Could you check a few things on this model? Use its own coordinates, in mm. A direction names the side the tool comes from. Coordinates: 2 decimals unless noted, no trailing zeros. Order: outer loops, then holes, each group sorted by start corner. A loop starts at its lowest first (then second) coordinate and runs counter-clockwise, first axis right, second up. Notation, with made-up numbers: (-8, -32) -> (0, -32) arc R25 ccw to (0, -14) -> close; hole circle Ø2 at (27.5, 2). An arc over 180 degrees is marked (long way). Use a Markdown table: item, result. Add a question column.
1) If we section it at B-B (z = -1.5): Write out the boundary of the cut face in (x, y).
2) If we section it at D-D (y = 1): Give the number of separate pieces and of enclosed holes in the cut face, plus the area to 3 significant figures.
3) Which directions (+Z, -Z, +X, -X, +Y, -Y) give clear straight access to the entire face, cutting with the end or side of a thin tool? Please do faces 1 (the flat face through (-69, 0, -35)), 2 (the flat face through (-49.5, 0, 15.3)), 3 (the flat face through (-50, -1, -42.716)).
4) If I drill on L1, parallel to Z at x = -29.5, y = 6.75; L2, parallel to Y at x = -40.5, z = -28.5; L3, parallel to X at y = 5, z = -32.5, over which ranges is the centre line in solid material (lowest first)? Write a range as [from, to].
5) If we section it at A-A (y = 10.5): Write out the boundary of the cut face in (x, z).
6) Will these pins go through, and if not, where does the flat tip stop? pin 1 Ø0.8 at (x, z) = (-50, 7.5) entering from +Y; pin 2 Ø6 at (x, y) = (-69, 5.5) entering from -Z; pin 3 Ø2 at (x, z) = (-49, 13.5) entering from +Y.
7) Thinking about a two-plate mould opening in X: for faces 4 (the flat face through (-69.4, 23, -33.9)), 5 (the cylindrical face through (-30.227, 11.339, -36.308)), 6 (the cylindrical face through (-52.64, 13.37, 6.98)), 7 (the cylindrical face through (-48.227, 11.339, 7.521)), which applies, +X half, -X half, draft (parallel to the pull), parting line (faces both ways), or undercut?
8) If we section it at C-C (x = -40.5): Write out the boundary of the cut face in (y, z).
```python
from build123d import *

# Parameters (mm, degrees)
SKETCH1_R           = 3.25
SKETCH1_R_2         = 1.25
BOSS_EXTRUDE1_DEPTH = 2
SKETCH1_3_R         = 3.25
SKETCH1_3_R_2       = 1.25
BOSS_EXTRUDE2_DEPTH = 23
FILLET1_R           = 4


with BuildPart() as part:
    # Sketch1 → Boss-Extrude1 (new body)
    # profile 1 of 7: a face of its own
    with BuildSketch(Plane(origin=(0, 0, 0), x_dir=(1, 0, 0), z_dir=(0, 1, 0))):
        with BuildLine():
            Line((-22.61799674, 34.235492608), (-44.003393626, -12.854176105))
            ThreePointArc((-44.003393626, -12.854176105), (-49.466422466, -16.373185197), (-54.929451307, -12.854176105))
            Line((-54.929451307, -12.854176105), (-76.314848193, 34.235492608))
            ThreePointArc((-76.314848193, 34.235492608), (-75.89592212, 39.96564145), (-70.851819352, 42.716483516))
            Line((-70.851819352, 42.716483516), (-28.08102558, 42.716483516))
            ThreePointArc((-28.08102558, 42.716483516), (-23.036922813, 39.96564145), (-22.61799674, 34.235492608))
        make_face()
        with Locations((-49.466422466, -7.683516484)):
            Circle(SKETCH1_R, mode=Mode.SUBTRACT)
        with Locations((-29.466422466, 35.316483516)):
            Circle(SKETCH1_R, mode=Mode.SUBTRACT)
        with Locations((-69.466422466, 35.316483516)):
            Circle(SKETCH1_R, mode=Mode.SUBTRACT)
    # profile 2 of 7: a face of its own
    with BuildSketch(Plane(origin=(0, 0, 0), x_dir=(1, 0, 0), z_dir=(0, 1, 0))):
        with Locations((-69.466422466, 35.316483516)):
            Circle(SKETCH1_R)
        with Locations((-69.466422466, 35.316483516)):
            Circle(SKETCH1_R_2, mode=Mode.SUBTRACT)
    # profile 3 of 7: a face of its own
    with BuildSketch(Plane(origin=(0, 0, 0), x_dir=(1, 0, 0), z_dir=(0, 1, 0))):
        with Locations((-69.466422466, 35.316483516)):
            Circle(SKETCH1_R_2)
    # profile 4 of 7: a face of its own
    with BuildSketch(Plane(origin=(0, 0, 0), x_dir=(1, 0, 0), z_dir=(0, 1, 0))):
        with Locations((-29.466422466, 35.316483516)):
            Circle(SKETCH1_R)
        with Locations((-29.466422466, 35.316483516)):
            Circle(SKETCH1_R_2, mode=Mode.SUBTRACT)
    # profile 5 of 7: a face of its own
    with BuildSketch(Plane(origin=(0, 0, 0), x_dir=(1, 0, 0), z_dir=(0, 1, 0))):
        with Locations((-29.466422466, 35.316483516)):
            Circle(SKETCH1_R_2)
    # profile 6 of 7: a face of its own
    with BuildSketch(Plane(origin=(0, 0, 0), x_dir=(1, 0, 0), z_dir=(0, 1, 0))):
        with Locations((-49.466422466, -7.683516484)):
            Circle(SKETCH1_R)
        with Locations((-49.466422466, -7.683516484)):
            Circle(SKETCH1_R_2, mode=Mode.SUBTRACT)
    # profile 7 of 7: a face of its own
    with BuildSketch(Plane(origin=(0, 0, 0), x_dir=(1, 0, 0), z_dir=(0, 1, 0))):
        with Locations((-49.466422466, -7.683516484)):
            Circle(SKETCH1_R_2)
    extrude(amount=-BOSS_EXTRUDE1_DEPTH)

    # Sketch1_3 → Boss-Extrude2 (add)
    # profile 1 of 3: a face of its own
    with BuildSketch(Plane(origin=(0, 0, 0), x_dir=(1, 0, 0), z_dir=(0, 1, 0))):
        with Locations(Location((-49.466422466, -7.683516484, 0), (0, 0, 270))):
            Circle(SKETCH1_3_R)
        with Locations(Location((-49.466422466, -7.683516484, 0), (0, 0, 270))):
            Circle(SKETCH1_3_R_2, mode=Mode.SUBTRACT)
    # profile 2 of 3: a face of its own
    with BuildSketch(Plane(origin=(0, 0, 0), x_dir=(1, 0, 0), z_dir=(0, 1, 0))):
        with Locations(Location((-29.466422466, 35.316483516, 0), (0, 0, 270))):
            Circle(SKETCH1_3_R)
        with Locations(Location((-29.466422466, 35.316483516, 0), (0, 0, 270))):
            Circle(SKETCH1_3_R_2, mode=Mode.SUBTRACT)
    # profile 3 of 3: a face of its own
    with BuildSketch(Plane(origin=(0, 0, 0), x_dir=(1, 0, 0), z_dir=(0, 1, 0))):
        with Locations(Location((-69.466422466, 35.316483516, 0), (0, 0, 270))):
            Circle(SKETCH1_3_R)
        with Locations(Location((-69.466422466, 35.316483516, 0), (0, 0, 270))):
            Circle(SKETCH1_3_R_2, mode=Mode.SUBTRACT)
    extrude(amount=BOSS_EXTRUDE2_DEPTH)

    # Fillet1
    fillet1_edges = [part.edges().sort_by_distance(p)[0] for p in [
        (-69.466422466, 0, -38.566483516),
        (-29.466422466, 0, -38.566483516),
        (-49.466422466, 0, 4.433516484),
    ]]
    fillet(fillet1_edges, radius=FILLET1_R)


solid = part.part
```
Answer sheet:
| question | item | result |
|---|---|---|
| 1 | outline | (-61.45, -2) -> (-37.48, -2) -> (-37.48, 0) -> (-61.45, 0) -> close |
| 2 | separate pieces | 3 |
| 2 | enclosed holes | 3 |
| 2 | area | 185 mm2 |
| 3 | face 1 | +Y |
| 3 | face 2 | +Z, +Y |
| 3 | face 3 | -Z, +X, -X, +Y, -Y |
| 4 | L1 | [-38.57, -36.57], [-34.07, -32.07] |
| 4 | L2 | [-2, 0] |
| 4 | L3 | [-71.09, -67.84], [-31.09, -27.84] |
| 5 | outline | circle Ø6.5 at (-69.47, -35.32); circle Ø6.5 at (-49.47, 7.68); circle Ø6.5 at (-29.47, -35.32); hole circle Ø2.5 at (-69.47, -35.32); hole circle Ø2.5 at (-49.47, 7.68); hole circle Ø2.5 at (-29.47, -35.32) |
| 6 | pin 1 | y = 0 |
| 6 | pin 2 | z = -38.85 |
| 6 | pin 3 | y = 0.81 |
| 7 | face 4 | draft |
| 7 | face 5 | undercut |
| 7 | face 6 | parting line |
| 7 | face 7 | undercut |
| 8 | outline | (-2, -42.72) -> (0, -42.72) -> (0, 5.14) -> (-2, 5.14) -> close |
